```python
from build123d import *

# Parameters (mm, degrees)
F1_DEPTH = 30
F3_D     = 6.6
F5_D     = 6.6
F6_D     = 4.2
F6_DEPTH = 14
F6_TIP   = 1.2618073


with BuildPart() as f1:
    # F0 (on Front) → F1 (new body)
    with BuildSketch(Plane.XZ):
        Polygon((8, 48), (0, 48), (0, 0), (26, 0), (26, 6), (8, 6), align=None)
    extrude(amount=F1_DEPTH)

    # F3 (through all)
    with Locations(Plane(origin=(0, 0, 0), x_dir=(0, -1, 0), z_dir=(-1, 0, 0))):
        with Locations((22, 38)):
            Hole(F3_D / 2)

    # F5 (through all)
    with Locations(Plane(origin=(0, 0, 0), x_dir=(1, 0, 0), z_dir=(0, 0, -1))):
        with Locations((18, 15)):
            Hole(F5_D / 2)

    # F6
    with Locations(Plane(origin=(0, 0, 0), x_dir=(1, 0, 0), z_dir=(0, 0, -1))):
        with Locations((4, 4), (4, 19)):
            Hole(F6_D / 2, depth=F6_DEPTH)
            with Locations((0, 0, -(F6_DEPTH + F6_TIP / 2))):  # 118° drill point
                Cone(0, F6_D / 2, F6_TIP, mode=Mode.SUBTRACT)


solid = f1.part
```
The model under review builds one solid part; all positions refer to its coordinate system, in mm. A direction names the side the tool comes from. Round coordinates to 2 decimals unless told otherwise and drop trailing zeros. Write each loop counter-clockwise with the first axis right and the second up, starting at its lowest first coordinate (ties: lowest second). Pieces come first, ordered by that corner, then holes. Notation, with made-up numbers: (42.5, 87) - (53.5, 87) arc R29 cw to (53.5, 107) - close; hole circle Ø2 at (54.25, 68). An arc over 180 degrees is marked (long way). Use one line per item in the form item = value.
Q1. Consider section C-C (y = -7.5). State the section outline as (x, z) points.
Answer key:
outline = (0, 0) - (26, 0) - (26, 6) - (8, 6) - (8, 48) - (0, 48) - close
Q2. Tool access review of faces 1 (the flat face through (0, -15, 24)), 2 (the flat face through (17, -11, 6)), 3 (the cylindrical face through (5.666, -2.722, 7.098)): name each direction out of +Z, -Z, +X, -X, +Y, -Y from which nothing blocks a thin tool from reaching the whole face with its end or side.
Answer key:
face_1 = +Z, -Z, -X, +Y, -Y
face_2 = +Z, +X, +Y, -Y
face_3 = -Z
Q3. Consider section A-A (x = 18). State the section outline as (y, z) points, and give its area (3 significant figures).
Answer key:
outline = (-30, 0) - (-18.3, 0) - (-18.3, 6) - (-30, 6) - close; (-11.7, 0) - (0, 0) - (0, 6) - (-11.7, 6) - close
area = 140 mm2
Q4. For line 1 (Y direction, x = 4, z = 10.75); line 2 (Y direction, x = 18, z = 1.45); line 3 (Z direction, x = 12.5, y = -1.75), list the stretches that pass through material, from the lowest coordinate up. Write a range as [from, to].
Answer key:
line_1 = [-30, -21.1], [-16.9, -6.1], [-1.9, 0]
line_2 = [-30, -18.3], [-11.7, 0]
line_3 = [0, 6]
Q5. Consider section B-B (y = -15). State the section outline as (x, z) points, and give its area (3 significant figures).
Answer key:
outline = (0, 0) - (14.7, 0) - (14.7, 6) - (8, 6) - (8, 48) - (0, 48) - close; (21.3, 0) - (26, 0) - (26, 6) - (21.3, 6) - close
area = 452 mm2
Q6. Insertion check: pin 1 Ø4 at (x, y) = (21, -16) entering from +Z; pin 2 Ø3.5 at (x, y) = (4, -19) entering from -Z; pin 3 Ø8 at (x, y) = (12, -16.5) entering from -Z; pin 4 Ø9 at (y, z) = (-15, 32.5) entering from +X. Each pin has a flat end and moves straight along its axis. Give the tip position at first contact, or say it passes through.
Answer key:
pin_1 = 6
pin_2 = 14.21
pin_3 = 0
pin_4 = 8
Q7. Consider section D-D (z = 18). State the section outline as (x, y) points, and give its area (3 significant figures).
Answer key:
outline = (0, -30) - (8, -30) - (8, 0) - (0, 0) - close
area = 240 mm2
Q8. Draft analysis for pull direction Y (two halves, no side actions). For faces 4 (the conical face through (4.2, -4.31, 15.04)), 5 (the flat face through (13, -15, 0)), 6 (the flat face through (7, 0, 19)), state which applies: +Y half, -Y half, draft (parallel to the pull), parting line (faces both ways), or undercut.
Answer key:
face_4 = undercut
face_5 = draft
face_6 = +Y half
